Part model, mm, in its own coordinate system. A direction names the side the tool comes from. Round coordinates to 2 decimals unless told otherwise and drop trailing zeros. Write each loop counter-clockwise with the first axis right and the second up, starting at its lowest first coordinate (ties: lowest second). Pieces come first, ordered by that corner, then holes.
1) Saw through at A-A on y = 5.25. Write the cut outline in (x, z).
2) Flat gauge pins, fed straight in: pin 1 (4.5 mm diameter, centred on y = 16.5, z = -9.5, fed in from +X); pin 2 (4 mm diameter, centred on y = 17.5, z = -10, fed in from +X); pin 3 (8 mm diameter, centred on x = 11.5, z = -3.5, fed in from +Y). Where does each tip first touch, or does it go through?
3) Saw through at D-D on y = 17.5. Write the cut outline in (x, z), and give its area (3 significant figures).
4) Saw through at C-C on z = -10. Write the cut outline in (x, y).
5) Saw through at B-B on x = 11.25. Write the cut outline in (y, z).
6) Which spindle directions (+Z, -Z, +X, -X, +Y, -Y) get a long thin tool onto all of the face, cutting with end or side? Do faces 4 (the flat face through (8, 5, -16)), 5 (the flat face through (6, 10, -20)), 6 (the flat face through (6.5, 21, -10)). Say none if no direction does.
7) Drill centre lines: L1, parallel to Y at x = 2, z = -10; L2, parallel to Y at x = 11.75, z = -8; L3, parallel to Y at x = 5.25, z = -7.5. Where is each one in solid material? Low to high.
8) Pull direction Y, two halves, no side cores. Call faces 1 (the flat face through (6, 10, 0)), 2 (the flat face through (8, 3.5, -10)), 3 (the flat face through (8, 0, -10)): +Y half, -Y half, draft (parallel to the pull), parting line (faces both ways), or undercut.
Autodesk Inventor part; units mm, degrees
ref_plane "YZ Plane" through (0, 0, 0) normal (1, 0, 0) x (0, 1, 0)
ref_plane "XZ Plane" through (0, 0, 0) normal (0, 1, 0) x (-1, 0, 0)
ref_plane "XY Plane" through (0, 0, 0) normal (0, 0, 1) x (1, 0, 0)
sketch "Sketch1" plane through (0, 0, 0) normal (1, 0, 0) x (0, 1, 0)
  line L0 (0, 0) -> (25, 0)
  line L1 (25, 0) -> (25, -20)
  line L2 (25, -20) -> (0, -20)
  line L3 (0, -20) -> (0, 0)
  line L4 (3.5, -4) -> (6.5, -4)
  line L5 (6.5, -4) -> (6.5, -16)
  line L6 (6.5, -16) -> (3.5, -16)
  line L7 (3.5, -16) -> (3.5, -4)
  dimension "d0" = 25
  dimension "d1" = 20
  dimension "d2" = 3
  dimension "d3" = 12
extrude "Extrusion1" add sketch "Sketch1" along normal blind 6.5
sketch "Sketch2" plane through (6.5, 0, 0) normal (1, 0, 0) x (0, 0, -1)
  line L0 (0, 25) -> (0, 0)
  line L1 (20, 0) -> (20, 25)
  line L2 (0, 0) -> (20, 0)
  line L3 (20, 0) -> (20, 10)
  line L4 (20, 10) -> (0, 10)
  line L5 (0, 10) -> (0, 0)
  line L6 (4, 3.5) -> (4, 6.5)
  line L7 (4, 6.5) -> (16, 6.5)
  line L8 (4, 3.5) -> (16, 3.5)
  line L9 (16, 3.5) -> (16, 6.5)
  line L10 (16, 6.5) -> (4, 6.5)
  line L11 (4, 6.5) -> (4, 3.5)
  dimension "d6" = 10
extrude "Extrusion2" add sketch "Sketch2" along normal blind 10
sketch "Sketch3" plane through (6.5, 0, 0) normal (1, 0, 0) x (0, 0, -1)
  line L0 (20, 0) -> (20, 25) construction
  line L1 (0, 10) -> (0, 0) construction
  line L2 (20, 25) -> (0, 10) construction
  circle A0 centre (10, 17.5) radius 3.2
  dimension "d9" = 6.4
extrude "Extrusion3" cut sketch "Sketch3" against normal blind 10
properties part number "_3DPrint"
Completed:
1. outline: (0, -20) - (16.5, -20) - (16.5, -16) - (0, -16) - close; (0, -4) - (16.5, -4) - (16.5, 0) - (0, 0) - close
2. pin 1: stops at x = 6.5
2. pin 2: passes through
2. pin 3: stops at y = 10
3. outline: (0, -20) - (6.5, -20) - (6.5, -13.2) - (0, -13.2) - close; (0, -6.8) - (6.5, -6.8) - (6.5, 0) - (0, 0) - close
3. area: 88.4 mm2
4. outline: (0, 0) - (16.5, 0) - (16.5, 3.5) - (0, 3.5) - close; (0, 6.5) - (16.5, 6.5) - (16.5, 10) - (6.5, 10) - (6.5, 14.3) - (0, 14.3) - close; (0, 20.7) - (6.5, 20.7) - (6.5, 25) - (0, 25) - close
5. outline: (0, -20) - (10, -20) - (10, 0) - (0, 0) - close; hole (3.5, -16) - (6.5, -16) - (6.5, -4) - (3.5, -4) - close
6. face 4: +X, -X
6. face 5: -Z, +X, -X, +Y, -Y
6. face 6: +Z, -Z, +X, +Y
7. L1: y = 0 to 3.5, 6.5 to 14.3, 20.7 to 25
7. L2: y = 0 to 3.5, 6.5 to 10
7. L3: y = 0 to 3.5, 6.5 to 15.5, 19.5 to 25
8. face 1: draft
8. face 2: undercut
8. face 3: -Y half
